The listing builds one solid part. Answer for the finished solid, in the listing's coordinates (mm). A direction names the side the tool comes from. Give positions to 0.01 mm unless a question says otherwise; leave off trailing zeros. Loops run counter-clockwise (first coordinate to the right, second up) from the corner with the lowest first, then second, coordinate; pieces in that order, holes last. Notation, with made-up numbers: (-38.75, -11.75) - (-15.75, -11.75) arc R17 cw to (-15.75, 11.25) - close; hole circle Ø1 at (7.25, 35.5). An arc over 180 degrees is marked (long way). Answer as CSV lines item,"result". Start each with the question number.
1) For faces 5 (the face through (10, 3, 0)), 6 (the face through (33.504, -0.346, 1.377)), 7 (the face through (33.63, 3.36, -1.39)), 8 (the face through (2.37, -0.768, 1.394)), determine the directions among +Z, -Z, +X, -X, +Y, -Y from which every point of the face is accessible in a straight line to the end or side of a thin tool.
2) Flat-ended cylindrical pins translate along their axes: pin 1 (3 mm diameter, centred on x = 0, z = 0, fed in from +Y); pin 2 (2 mm diameter, centred on y = 0, z = -1.5, fed in from +X); pin 3 (2 mm diameter, centred on x = 20, y = 2, fed in from -Z); pin 4 (1 mm diameter, centred on y = 0, z = 2, fed in from -X). Find the tip coordinate at first contact, or state that the pin passes through.
3) For a pull along Z with two mould halves and no side action, classify faces 1 (the face through (1.4, 0.5, 1.2)), 2 (the face through (-5, 1, 0)), 3 (the face through (38.37, 1.56, -1.38)), 4 (the face through (33.488, -0.473, 0.018)) as pulls with the +Z half, pulls with the -Z half, needs draft (parallel to the pull), parting line crosses it, or undercut.
4) A cutting plane is placed at A-A (y = 1.5). Determine the outline of the cut face in (x, z) (3 decimals), and give its area (3 significant figures).
5) A cutting plane is placed at B-B (x = 36). Determine the outline of the cut face in (y, z).
6) Find the intervals of material crossed by line 1 along X through (y, z) = (1.5, -0.3); line 2 along Y through (x, z) = (36, 0.1); line 3 along Z through (x, y) = (23, 1.8), in increasing order.
7) A cutting plane is placed at C-C (x = 29). Determine the outline of the cut face in (y, z).
8) A cutting plane is placed at D-D (z = 0.5). Give the number of separate pieces and of enclosed holes in the cut face, and give its area (3 significant figures).
```python
from build123d import *

# Parameters (mm, degrees)
EXTRUDE_1_DEPTH     = 3
EXTRUDE_START       = 1.5
SKETCH_2_R          = 2.5
EXTRUDE_2_DEPTH     = 3
CUT_EXTRUDE_START   = -1.5
SKETCH_3_R          = 1
CUT_EXTRUDE_1_DEPTH = 3
EXTRUDE_3_DEPTH     = 3
EXTRUDE_4_DEPTH     = 3
SKETCH_7_R          = 5.01204864
EXTRUDE_5_DEPTH     = 2
CUT_EXTRUDE_START_2 = -2
CUT_EXTRUDE_2_DEPTH = 2.5
CUT_EXTRUDE_START_3 = 3
SKETCH_9_R          = 1.625
CUT_EXTRUDE_3_DEPTH = 5
CHAMFER_3_SIZE      = 0.25


with BuildPart() as part:
    # 草图1 → 凸台-拉伸1 (new body)
    with BuildSketch(Plane(origin=(0, 0, 0), x_dir=(1, 0, 0), z_dir=(0, 1, 0))):
        with BuildLine():
            Line((36, -1.5), (36, 1.5))
            Line((36, 1.5), (4.769696007, 1.5))
            ThreePointArc((4.769696007, 1.5), (-5, 0), (4.769696007, -1.5))
            Line((4.769696007, -1.5), (36, -1.5))
        make_face()
    extrude(amount=EXTRUDE_1_DEPTH)

    # 草图2 → 凸台-拉伸2 (add)
    with BuildSketch(Plane.XY.offset(EXTRUDE_START)):
        with Locations((36, 1.5)):
            Circle(SKETCH_2_R)
    extrude(amount=-EXTRUDE_2_DEPTH)

    # 草图3 → 切除-拉伸1 (cut)
    with BuildSketch(Plane.XY.offset(CUT_EXTRUDE_START)):
        with Locations(Location((36, 1.5, 0), (0, 0, 180))):
            Circle(SKETCH_3_R)
    extrude(amount=CUT_EXTRUDE_1_DEPTH, mode=Mode.SUBTRACT)

    # 草图5 → 凸台-拉伸3 (add)
    with BuildSketch(Plane.XY.offset(EXTRUDE_START)):
        with BuildLine():
            ThreePointArc((35.421854812, 3.932231104), (34.629244055, 3.590700395), (34, 3))
            Line((34, 3), (31.5, 3))
            Line((31.5, 3), (35.421854812, 3.932231104))
        make_face()
        with BuildLine():
            ThreePointArc((34, 0), (34.629244055, -0.590700395), (35.421854812, -0.932231104))
            Line((35.421854812, -0.932231104), (31.5, 0))
            Line((31.5, 0), (34, 0))
        make_face()
    extrude(amount=-EXTRUDE_3_DEPTH)

    # 草图6 → 凸台-拉伸4 (add)
    with BuildSketch(Plane(origin=(0, 0, 0), x_dir=(1, 0, 0), z_dir=(0, 1, 0))):
        with BuildLine():
            ThreePointArc((4.769696007, 1.5), (3.662773496, 3.40354085), (1.845456766, 4.646965604))
            Line((1.845456766, 4.646965604), (9.769696007, 1.5))
            Line((9.769696007, 1.5), (4.769696007, 1.5))
        make_face()
        with BuildLine():
            ThreePointArc((1.845456766, -4.646965604), (3.662773496, -3.40354085), (4.769696007, -1.5))
            Line((4.769696007, -1.5), (9.769696007, -1.5))
            Line((9.769696007, -1.5), (1.845456766, -4.646965604))
        make_face()
    extrude(amount=EXTRUDE_4_DEPTH)

    # 草图7 → 凸台-拉伸5 (add)
    with BuildSketch(Plane(origin=(0, 0, 0), x_dir=(1, 0, 0), z_dir=(0, 1, 0))):
        with Locations(Location((0, 0, 0), (0, 0, 270))):
            Circle(SKETCH_7_R)
    extrude(amount=-EXTRUDE_5_DEPTH)

    # 草图8 → 切除-拉伸2 (cut)
    with BuildSketch(Plane(origin=(0, 0, 0), x_dir=(1, 0, 0), z_dir=(0, 1, 0)).offset(CUT_EXTRUDE_START_2)):
        Polygon((3.175426481, 0), (1.58771324, 2.75), (-1.58771324, 2.75), (-3.175426481, 0), (-1.58771324, -2.75), (1.58771324, -2.75), align=None)
    extrude(amount=CUT_EXTRUDE_2_DEPTH, mode=Mode.SUBTRACT)

    # 草图9 → 切除-拉伸3 (cut)
    with BuildSketch(Plane(origin=(0, 0, 0), x_dir=(1, 0, 0), z_dir=(0, 1, 0)).offset(CUT_EXTRUDE_START_3)):
        with Locations(Location((0, 0, 0), (0, 0, 270))):
            Circle(SKETCH_9_R)
    extrude(amount=-CUT_EXTRUDE_3_DEPTH, mode=Mode.SUBTRACT)

    # 倒角3
    # the kernel refuses this chamfer: 0.25 mm, written as the material it adds along each edge
    with BuildSketch(Plane(origin=(0, 0, 0), x_dir=(0.31362035772557234, 0, 0.949548456488706), z_dir=(-0.949548456488706, 0, 0.31362035772557234))) as chamfer_3_piece_1_section:
        Polygon((5.01204864 + CHAMFER_3_SIZE, 0), (5.01204864, -CHAMFER_3_SIZE), (5.01204864, 0), align=None)
    chamfer_3_piece_1 = revolve(axis=Axis((0, 0, 0), (0, 1, 0)), revolution_arc=143.444907743, mode=Mode.PRIVATE)
    chamfer_3_piece_1 = split(chamfer_3_piece_1, bisect_by=Plane(origin=(1.845456766, 0, 4.646965604), z_dir=(-0.3690913531117439, 0, -0.929393120836464)), keep=Keep.TOP, mode=Mode.PRIVATE)
    chamfer_3_piece_1 = split(chamfer_3_piece_1, bisect_by=Plane(origin=(1.845456766, 0, -4.646965604), z_dir=(-0.3690913531117441, 0, 0.9293931208364639)), keep=Keep.TOP, mode=Mode.PRIVATE)
    add(chamfer_3_piece_1)
    # the kernel refuses this chamfer: 0.25 mm, written as the material it takes off along each edge
    with BuildSketch(Plane(origin=(0, 3, 0), x_dir=(0, 0, 1), z_dir=(-1, 0, 0))) as chamfer_3_2_piece_1:
        Polygon((1.625 + CHAMFER_3_SIZE, 0), (1.625, -CHAMFER_3_SIZE), (1.625, 0), align=None)
    revolve(axis=Axis((0, 3, 0), (0, 1, 0)), mode=Mode.SUBTRACT)
    with BuildSketch(Plane(origin=(36, 1.5, 1.5), x_dir=(-1, 0, 0), z_dir=(0, 1, 0))) as chamfer_3_2_piece_2:
        Polygon((1 + CHAMFER_3_SIZE, 0), (1, -CHAMFER_3_SIZE), (1, 0), align=None)
    revolve(axis=Axis((36, 1.5, 1.5), (0, 0, 1)), mode=Mode.SUBTRACT)
    with BuildSketch(Plane(origin=(36, 1.5, -1.5), x_dir=(-1, 0, 0), z_dir=(0, 1, 0))) as chamfer_3_2_piece_3:
        Polygon((1, CHAMFER_3_SIZE), (1 + CHAMFER_3_SIZE, 0), (1, 0), align=None)
    revolve(axis=Axis((36, 1.5, -1.5), (0, 0, 1)), mode=Mode.SUBTRACT)
    with BuildSketch(Plane(origin=(36, 1.5, 1.5), x_dir=(-0.23125807505671483, -0.9728924414965218, 0), z_dir=(-0.9728924414965218, 0.23125807505671483, 0))) as chamfer_3_2_piece_4:
        Polygon((2.5 - CHAMFER_3_SIZE, 0), (2.5, -CHAMFER_3_SIZE), (2.5, 0), align=None)
    revolve(axis=Axis((36, 1.5, 1.5), (0, 0, 1)), revolution_arc=206.742302393, mode=Mode.SUBTRACT)
    with BuildSketch(Plane(origin=(32.142920747, 3, -1.5), x_dir=(0, 0, 1), z_dir=(-1, 0, 0))) as chamfer_3_2_piece_5_section:
        Polygon((CHAMFER_3_SIZE, 0), (0, -CHAMFER_3_SIZE), (0, 0), align=None)
    chamfer_3_2_piece_5 = extrude(amount=23.016145487, mode=Mode.PRIVATE)
    chamfer_3_2_piece_5 = split(chamfer_3_2_piece_5, bisect_by=Plane(origin=(32.15463621, 2.950713568, -1.449340307), z_dir=(-0.16352415307675153, 0.6879388427473303, -0.7071067811865444)), keep=Keep.TOP, mode=Mode.PRIVATE)
    chamfer_3_2_piece_5 = split(chamfer_3_2_piece_5, bisect_by=Plane(origin=(30.572849722, -1.253881896, 2.453528571), z_dir=(0.26098699866263353, 0.7071067811865455, -0.6571801781315938)), keep=Keep.TOP, mode=Mode.PRIVATE)
    add(chamfer_3_2_piece_5, mode=Mode.SUBTRACT)
    with BuildSketch(Plane(origin=(30.874507265, 2.851319386, -1.5), x_dir=(0, 0, 1), z_dir=(0.9728924414965218, 0.231258075056715, 0))) as chamfer_3_2_piece_6_section:
        Polygon((CHAMFER_3_SIZE, 0), (0, CHAMFER_3_SIZE), (0, 0), align=None)
    chamfer_3_2_piece_6 = extrude(amount=4.674049621, mode=Mode.PRIVATE)
    chamfer_3_2_piece_6 = split(chamfer_3_2_piece_6, bisect_by=Plane(origin=(30.874507265, 2.800659693, -1.449340307), z_dir=(0, 0.7071067811865476, -0.7071067811865476)), keep=Keep.TOP, mode=Mode.PRIVATE)
    add(chamfer_3_2_piece_6, mode=Mode.SUBTRACT)
    with BuildSketch(Plane(origin=(30.874507265, 2.851319386, 1.5), x_dir=(0.23125807505671495, -0.9728924414965217, 0), z_dir=(0.9728924414965218, 0.231258075056715, 0))) as chamfer_3_2_piece_7_section:
        Polygon((CHAMFER_3_SIZE, 0), (0, CHAMFER_3_SIZE), (0, 0), align=None)
    chamfer_3_2_piece_7 = extrude(amount=4.674049621, mode=Mode.PRIVATE)
    chamfer_3_2_piece_7 = split(chamfer_3_2_piece_7, bisect_by=Plane(origin=(30.874507265, 2.800659693, 1.449340307), z_dir=(0, 0.7071067811865476, 0.7071067811865476)), keep=Keep.TOP, mode=Mode.PRIVATE)
    add(chamfer_3_2_piece_7, mode=Mode.SUBTRACT)
    with BuildSketch(Plane(origin=(36, 1.5, -1.5), x_dir=(-0.23125807505671483, 0.9728924414965218, 0), z_dir=(-0.9728924414965218, -0.23125807505671483, 0))) as chamfer_3_2_piece_8:
        Polygon((2.5, -CHAMFER_3_SIZE), (2.5 - CHAMFER_3_SIZE, 0), (2.5, 0), align=None)
    revolve(axis=Axis((36, 1.5, -1.5), (0, 0, -1)), revolution_arc=206.742302393, mode=Mode.SUBTRACT)
    with BuildSketch(Plane(origin=(32.142920747, 0, -1.5), x_dir=(0, 0, 1), z_dir=(-1, 0, 0))) as chamfer_3_2_piece_9_section:
        Polygon((CHAMFER_3_SIZE, 0), (0, CHAMFER_3_SIZE), (0, 0), align=None)
    chamfer_3_2_piece_9 = extrude(amount=23.016145487, mode=Mode.PRIVATE)
    chamfer_3_2_piece_9 = split(chamfer_3_2_piece_9, bisect_by=Plane(origin=(29.095051535, 0, 6.174708862), z_dir=(0.3690913531117441, 0, -0.9293931208364639)), keep=Keep.TOP, mode=Mode.PRIVATE)
    chamfer_3_2_piece_9 = split(chamfer_3_2_piece_9, bisect_by=Plane(origin=(32.15463621, 0.049286432, -1.449340307), z_dir=(-0.16352415307675064, -0.6879388427473256, -0.7071067811865488)), keep=Keep.TOP, mode=Mode.PRIVATE)
    add(chamfer_3_2_piece_9, mode=Mode.SUBTRACT)
    with BuildSketch(Plane(origin=(35.421854812, -0.932231104, 1.5), x_dir=(0.23125807505671522, 0.9728924414965215, 0), z_dir=(-0.9728924414965217, 0.23125807505671525, 0))) as chamfer_3_2_piece_10_section:
        Polygon((CHAMFER_3_SIZE, 0), (0, CHAMFER_3_SIZE), (0, 0), align=None)
    chamfer_3_2_piece_10 = extrude(amount=4.674049621, mode=Mode.PRIVATE)
    chamfer_3_2_piece_10 = split(chamfer_3_2_piece_10, bisect_by=Plane(origin=(35.421854812, -0.341115552, 0.908884448), z_dir=(0, -0.7071067811865476, 0.7071067811865476)), keep=Keep.TOP, mode=Mode.PRIVATE)
    add(chamfer_3_2_piece_10, mode=Mode.SUBTRACT)
    with BuildSketch(Plane(origin=(35.421854812, -0.932231104, -1.5), x_dir=(0, 0, 1), z_dir=(-0.9728924414965217, 0.23125807505671525, 0))) as chamfer_3_2_piece_11_section:
        Polygon((CHAMFER_3_SIZE, 0), (0, CHAMFER_3_SIZE), (0, 0), align=None)
    chamfer_3_2_piece_11 = extrude(amount=4.674049621, mode=Mode.PRIVATE)
    chamfer_3_2_piece_11 = split(chamfer_3_2_piece_11, bisect_by=Plane(origin=(35.421854812, -0.341115552, -0.908884448), z_dir=(0, -0.7071067811865476, -0.7071067811865476)), keep=Keep.TOP, mode=Mode.PRIVATE)
    add(chamfer_3_2_piece_11, mode=Mode.SUBTRACT)
    with BuildSketch(Plane(origin=(0, 3, 0), x_dir=(0.36909135311174435, 0, -0.9293931208364636), z_dir=(0.9293931208364636, 0, 0.36909135311174435))) as chamfer_3_2_piece_12:
        Polygon((5 - CHAMFER_3_SIZE, 0), (5, -CHAMFER_3_SIZE), (5, 0), align=None)
    revolve(axis=Axis((0, 3, 0), (0, 1, 0)), revolution_arc=223.319179184, mode=Mode.SUBTRACT)
    with BuildSketch(Plane(origin=(1.845456766, 3, -4.646965604), x_dir=(-0.3690913531117441, 0, 0.9293931208364639), z_dir=(0.9293931208364639, 0, 0.3690913531117441))) as chamfer_3_2_piece_13_section:
        Polygon((CHAMFER_3_SIZE, 0), (0, CHAMFER_3_SIZE), (0, 0), align=None)
    chamfer_3_2_piece_13 = extrude(amount=9.169171979, mode=Mode.PRIVATE)
    chamfer_3_2_piece_13 = split(chamfer_3_2_piece_13, bisect_by=Plane(origin=(1.845456766, 1.301517198, -2.948482802), z_dir=(0, 0.7071067811865476, -0.7071067811865476)), keep=Keep.TOP, mode=Mode.PRIVATE)
    add(chamfer_3_2_piece_13, mode=Mode.SUBTRACT)
    with BuildSketch(Plane(origin=(9.12677526, 0, 1.5), x_dir=(0, 1, 0), z_dir=(1, 0, 0))) as chamfer_3_2_piece_14_section:
        Polygon((CHAMFER_3_SIZE, 0), (0, -CHAMFER_3_SIZE), (0, 0), align=None)
    chamfer_3_2_piece_14 = extrude(amount=23.016145487, mode=Mode.PRIVATE)
    chamfer_3_2_piece_14 = split(chamfer_3_2_piece_14, bisect_by=Plane(origin=(9.214359342, 0, 1.720541724), z_dir=(0.3690913531117439, 0, 0.929393120836464)), keep=Keep.TOP, mode=Mode.PRIVATE)
    chamfer_3_2_piece_14 = split(chamfer_3_2_piece_14, bisect_by=Plane(origin=(9.753945875, 2.638478895, -1.211994443), z_dir=(-0.16352415307675064, -0.6879388427473256, 0.7071067811865488)), keep=Keep.TOP, mode=Mode.PRIVATE)
    add(chamfer_3_2_piece_14, mode=Mode.SUBTRACT)
    with BuildSketch(Plane(origin=(9.12677526, 3, 1.5), x_dir=(0, -1, 0), z_dir=(1, 0, 0))) as chamfer_3_2_piece_15_section:
        Polygon((CHAMFER_3_SIZE, 0), (0, CHAMFER_3_SIZE), (0, 0), align=None)
    chamfer_3_2_piece_15 = extrude(amount=23.016145487, mode=Mode.PRIVATE)
    chamfer_3_2_piece_15 = split(chamfer_3_2_piece_15, bisect_by=Plane(origin=(9.753945875, 0.361521105, -1.211994443), z_dir=(-0.16352415307675153, 0.6879388427473303, 0.7071067811865444)), keep=Keep.TOP, mode=Mode.PRIVATE)
    chamfer_3_2_piece_15 = split(chamfer_3_2_piece_15, bisect_by=Plane(origin=(9.124430882, 2.993648244, 1.494096722), z_dir=(0.2609869986626325, 0.7071067811865481, 0.6571801781315915)), keep=Keep.TOP, mode=Mode.PRIVATE)
    add(chamfer_3_2_piece_15, mode=Mode.SUBTRACT)
    with BuildSketch(Plane(origin=(10.367222127, 3, 1.262703512), x_dir=(-0.3690913531117439, 0, -0.929393120836464), z_dir=(-0.9293931208364639, 0, 0.36909135311174385))) as chamfer_3_2_piece_16_section:
        Polygon((CHAMFER_3_SIZE, 0), (0, CHAMFER_3_SIZE), (0, 0), align=None)
    chamfer_3_2_piece_16 = extrude(amount=9.169171979, mode=Mode.PRIVATE)
    chamfer_3_2_piece_16 = split(chamfer_3_2_piece_16, bisect_by=Plane(origin=(10.367222127, 2.993648244, 1.256351756), z_dir=(0, 0.7071067811865476, 0.7071067811865476)), keep=Keep.TOP, mode=Mode.PRIVATE)
    add(chamfer_3_2_piece_16, mode=Mode.SUBTRACT)
    with BuildSketch(Plane(origin=(0, -2, 0), x_dir=(0, 0, 1), z_dir=(-1, 0, 0))) as chamfer_3_2_piece_17:
        Polygon((5.01204864, CHAMFER_3_SIZE), (5.01204864 - CHAMFER_3_SIZE, 0), (5.01204864, 0), align=None)
    revolve(axis=Axis((0, -2, 0), (0, 1, 0)), mode=Mode.SUBTRACT)


solid = part.part
```
Ans:
1,face 5,"+Z, -Z, -X, +Y"
1,face 6,"+Z, -Y"
1,face 7,"-Z, +Y"
1,face 8,"-Y"
2,pin 1,"through"
2,pin 2,"x = 38.44"
2,pin 3,"z = -1.5"
2,pin 4,"x = -4.78"
3,face 1,"undercut"
3,face 2,"parting line crosses it"
3,face 3,"pulls with the -Z half"
3,face 4,"needs draft"
4,outline,"(1.845, -4.647) - (9.77, -1.5) - (34.75, -1.5) - (35, -1.25) - (35, 1.25) - (34.75, 1.5) - (9.77, 1.5) - (1.845, 4.647) arc R5 ccw (long way) to start; (37, -1.25) - (37.25, -1.5) - (38.25, -1.5) - (38.5, -1.25) - (38.5, 1.25) - (38.25, 1.5) - (37.25, 1.5) - (37, 1.25) - close; hole circle Ø3.25 at (0, 0)"
4,area,"178 mm2"
5,outline,"(-1, -1.25) - (-0.75, -1.5) - (0.25, -1.5) - (0.5, -1.25) - (0.5, 1.25) - (0.25, 1.5) - (-0.75, 1.5) - (-1, 1.25) - close; (2.5, -1.25) - (2.75, -1.5) - (3.75, -1.5) - (4, -1.25) - (4, 1.25) - (3.75, 1.5) - (2.75, 1.5) - (2.5, 1.25) - close"
6,line 1,"-4.99 to -1.6, 1.6 to 35, 37 to 38.5"
6,line 2,"-1 to 0.5, 2.5 to 4"
6,line 3,"-1.5 to 1.5"
7,outline,"(0, -1.25) - (0.25, -1.5) - (2.75, -1.5) - (3, -1.25) - (3, 1.25) - (2.75, 1.5) - (0.25, 1.5) - (0, 1.25) - close"
8,separate pieces,"2"
8,enclosed holes,"1"
8,area,"132 mm2"
